Could you check a few things on this drawing? It's one solid part, dimensions in mm from its lowest x, y, z. Give positions to 0.01 mm unless a question says otherwise; leave off trailing zeros. Order: outer loops, then holes, each group sorted by start corner. A loop starts at its lowest first (then second) coordinate and runs counter-clockwise, first axis right, second up.
Item 1: I'm going to push a flat-ended pin straight in: pin 1 Ø5 at (x, y) = (23, 55) entering from -Z. Where does the tip first touch, or does it pass through?
Item 2: If I drill on line 1 along X through (y, z) = (88.25, 4); line 2 along Y through (x, z) = (472.5, 6.5); line 3 along Y through (x, z) = (312.5, 12), over which ranges is the centre line in solid material (lowest first)?
Item 3: I want a section at A-A, the plane x = 472.5. Write out the boundary of the cut face in (y, z), then the cut area to 3 significant figures.
Item 4: I want a section at B-B, the plane y = 120.5. Write out the boundary of the cut face in (x, z).
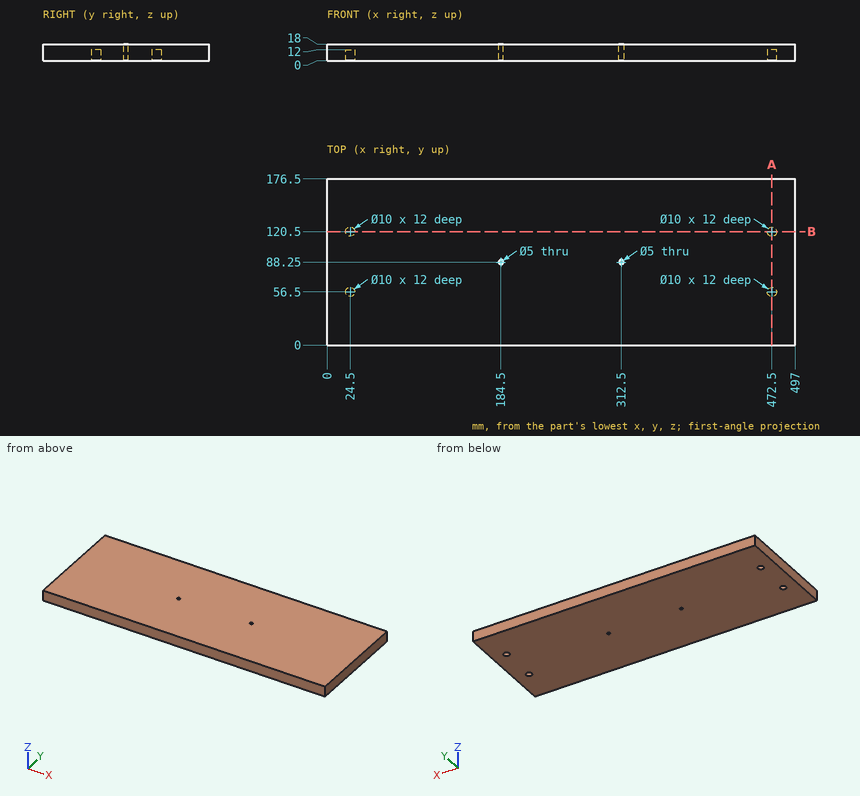
Results list:
1. pin 1: stops at z = 12
2. line 1: x = 0 to 182, 187 to 310, 315 to 497
2. line 2: y = 0 to 51.5, 61.5 to 115.5, 125.5 to 176.5
2. line 3: y = 0 to 85.75, 90.75 to 176.5
3. outline: (0, 0) - (51.5, 0) - (51.5, 12) - (61.5, 12) - (61.5, 0) - (115.5, 0) - (115.5, 12) - (125.5, 12) - (125.5, 0) - (176.5, 0) - (176.5, 18) - (0, 18) - close
3. area: 2,940 mm2
4. outline: (0, 0) - (19.5, 0) - (19.5, 12) - (29.5, 12) - (29.5, 0) - (467.5, 0) - (467.5, 12) - (477.5, 12) - (477.5, 0) - (497, 0) - (497, 18) - (0, 18) - close
